Autodesk Inventor part; units mm, degrees
ref_plane "YZ Plane" through (0, 0, 0) normal (1, 0, 0) x (0, 1, 0)
ref_plane "XZ Plane" through (0, 0, 0) normal (0, 1, 0) x (-1, 0, 0)
ref_plane "XY Plane" through (0, 0, 0) normal (0, 0, 1) x (1, 0, 0)
sketch "Sketch1" plane through (0, 0, 0) normal (0, 0, 1) x (1, 0, 0)
  line L0 (2.7, -6.25) -> (16.5, -6.25)
  line L1 (16.5, -6.25) -> (16.5, 0)
  line L2 (16.5, 0) -> (0, 0)
  line L3 (0, 0) -> (0, -2.5)
  line L4 (0, -2.5) -> (1.5, -2.5)
  line L5 (1.5, -2.5) -> (1.5, -12)
  line L6 (1.5, -12) -> (2.7, -12)
  line L7 (2.7, -12) -> (2.7, -6.25)
  dimension "d0" = 6.25
  dimension "d1" = 15
  dimension "d2" = 1.2
  dimension "d3" = 12
  dimension "d4" = 2.5
  dimension "d5" = 1.5
revolve "Revolution1" add sketch "Sketch1" angle 360 about axis through (16.5, 0, 0) along (-1, 0, 0)
sketch "Sketch2" plane through (1.5, 0, 0) normal (-1, 0, 0) x (0, 0, 1)
  circle A0 centre (0, 0) radius 9 construction
  circle A1 centre (0, -9) radius 1.6
  line L0 (0, -16.8) -> (0, 16.8)
  circle A2 centre (7.7942, 4.5) radius 1.6
  circle A3 centre (-7.7942, 4.5) radius 1.6
  dimension "d7" = 18
  dimension "d8" = 3.2
  dimension "d11" = 360
extrude "Extrusion1" cut sketch "Sketch2" against normal blind 1.2
sketch "Sketch3" plane through (0, 0, 0) normal (-1, 0, 0) x (0, 0, 1)
  circle A0 centre (0, 0) radius 2.5
  point P0 (0, 0)
extrude "Extrusion2" add sketch "Sketch3" along normal blind 1.5
sketch "Sketch4" plane through (1.5, 0, 0) normal (-1, 0, 0) x (0, 0, 1)
  circle A0 centre (0, 0) radius 5
  dimension "d17" = 10
extrude "Extrusion3" add sketch "Sketch4" along normal blind 1
properties part number "SRM-12-06A"
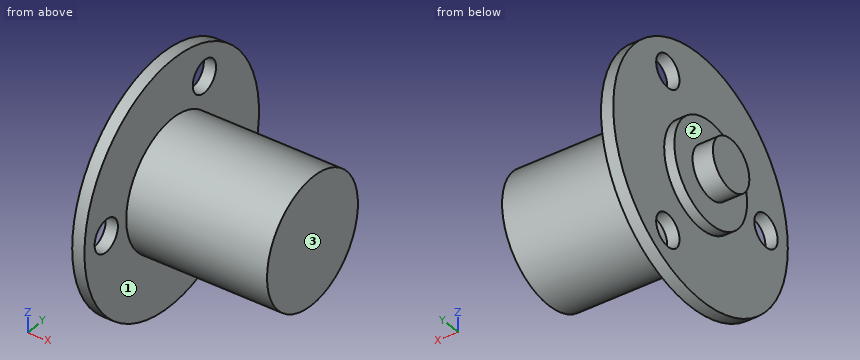
Design review of the part built by this model. Coordinates are the model's own, in mm. Face numbers are marked on the shaded views. A direction names the side the tool comes from. Coordinates: 2 decimals unless noted, no trailing zeros. Write each loop counter-clockwise with the first axis right and the second up, starting at its lowest first coordinate (ties: lowest second). Pieces come first, ordered by that corner, then holes.
1) Insertion check: pin 1 (3 mm diameter, centred on y = -9, z = 0, fed in from +X); pin 2 (6 mm diameter, centred on y = 1, z = 8.5, fed in from -X); pin 3 (6 mm diameter, centred on x = 7.5, y = -6.5, fed in from -Z); pin 4 (5 mm diameter, centred on x = 11, y = -3, fed in from +Z). Each pin has a flat end and moves straight along its axis. Give the tip position at first contact, or say it passes through.
2) Add section B-B (y = -9). Write out the cut boundary in (x, z).
3) Add section D-D (y = 4.5). Write out the cut boundary in (x, z), plus the area to 3 significant figures.
4) Add section C-C (y = 0). Write out the cut boundary in (x, z).
5) Add section A-A (z = 0). Write out the cut boundary in (x, y).
6) Machinability: for the marked faces 1, 2 and 3, which of the approach directions +Z, -Z, +X, -X, +Y, -Y give a long, thin tool a straight path to every point of the face, cutting with its end or side? Answer none if there is none.
7) To check wall thickness, follow L1, parallel to X at y = 9.25, z = 3.25; L2, parallel to X at y = 2.5, z = 3; L3, parallel to Z at x = 2.05, y = -9. State the ranges of each line that lie inside material, in increasing order.
Check result:
1. pin 1: passes through
1. pin 2: stops at x = 1.5
1. pin 3: stops at z = -5.18
1. pin 4: stops at z = 6.23
2. outline: (1.5, -7.94) - (2.7, -7.94) - (2.7, -1.6) - (1.5, -1.6) - close; (1.5, 1.6) - (2.7, 1.6) - (2.7, 7.94) - (1.5, 7.94) - close
3. outline: (0.5, -2.18) - (1.5, -2.18) - (1.5, -6.19) - (2.7, -6.19) - (2.7, -4.34) - (16.5, -4.34) - (16.5, 4.34) - (2.7, 4.34) - (2.7, 6.19) - (1.5, 6.19) - (1.5, 2.18) - (0.5, 2.18) - close; (1.5, -11.12) - (2.7, -11.12) - (2.7, -9.39) - (1.5, -9.39) - close; (1.5, 9.39) - (2.7, 9.39) - (2.7, 11.12) - (1.5, 11.12) - close
3. area: 143 mm2
4. outline: (-1.5, -2.5) - (0.5, -2.5) - (0.5, -5) - (1.5, -5) - (1.5, -12) - (2.7, -12) - (2.7, -6.25) - (16.5, -6.25) - (16.5, 6.25) - (2.7, 6.25) - (2.7, 12) - (1.5, 12) - (1.5, 5) - (0.5, 5) - (0.5, 2.5) - (-1.5, 2.5) - close
5. outline: (-1.5, -2.5) - (0.5, -2.5) - (0.5, -5) - (1.5, -5) - (1.5, -7.4) - (2.7, -7.4) - (2.7, -6.25) - (16.5, -6.25) - (16.5, 6.25) - (2.7, 6.25) - (2.7, 12) - (1.5, 12) - (1.5, 5) - (0.5, 5) - (0.5, 2.5) - (-1.5, 2.5) - close; (1.5, -12) - (2.7, -12) - (2.7, -10.6) - (1.5, -10.6) - close
6. face 1: +X
6. face 2: -X
6. face 3: +Z, -Z, +X, +Y, -Y
7. L1: x = 1.5 to 2.7
7. L2: x = 0.5 to 16.5
7. L3: z = -7.94 to -1.6, 1.6 to 7.94
